The model under review builds one solid part; all positions refer to its coordinate system, in mm. Round coordinates to 2 decimals unless told otherwise and drop trailing zeros. Order: outer loops, then holes, each group sorted by start corner. A loop starts at its lowest first (then second) coordinate and runs counter-clockwise, first axis right, second up. Notation, with made-up numbers: (12.25, -22.5) -> (71.25, -22.5) arc R19 ccw to (71.25, 9.5) -> close; hole circle Ø6 at (33.25, 60.5). An arc over 180 degrees is marked (long way). Use a Markdown table: item, result. Add a question column.
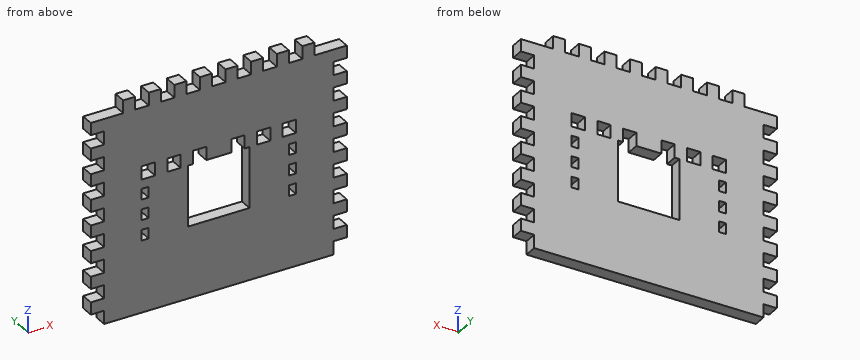
```python
from build123d import *

# Parameters (mm, degrees)
SKETCH1_W           = 127
SKETCH1_H           = 107.95
BOSS_EXTRUDE1_DEPTH = 6.35
SKETCH2_W           = 6.604
SKETCH2_H           = 6.604
CUT_EXTRUDE1_DEPTH  = 84.58153579
SKETCH3_W           = 3.429
SKETCH3_H           = 5.334
SKETCH3_W_2         = 6.604
SKETCH3_H_2         = 6.604
CUT_EXTRUDE4_DEPTH  = 84.58153579


with BuildPart() as part:
    # Sketch1 → Boss-Extrude1 (new body)
    with BuildSketch(Plane(origin=(0, 0, 0), x_dir=(1, 0, 0), z_dir=(0, 1, 0))):
        Rectangle(SKETCH1_W, SKETCH1_H)
    extrude(amount=BOSS_EXTRUDE1_DEPTH)

    # Sketch2 → Cut-Extrude1 (cut, through all)
    with BuildSketch(Plane.XZ):
        Polygon((-34.7345, 47.625), (-41.4655, 47.625), (-41.4655, 54.229), (-47.4345, 54.229), (-47.4345, 47.625), (-56.896, 47.625), (-63.5, 47.625), (-63.5, 54.229), (-63.5, 63.03162391), (63.5, 63.03162391), (63.5, 54.229), (63.5, 47.625), (56.896, 47.625), (47.4345, 47.625), (47.4345, 54.229), (41.4655, 54.229), (41.4655, 47.625), (34.7345, 47.625), (34.7345, 54.229), (28.7655, 54.229), (28.7655, 47.625), (22.0345, 47.625), (22.0345, 54.229), (16.0655, 54.229), (16.0655, 47.625), (9.3345, 47.625), (9.3345, 54.229), (3.3655, 54.229), (3.3655, 47.625), (-3.3655, 47.625), (-3.3655, 54.229), (-9.3345, 54.229), (-9.3345, 47.625), (-16.0655, 47.625), (-16.0655, 54.229), (-22.0345, 54.229), (-22.0345, 47.625), (-28.7655, 47.625), (-28.7655, 54.229), (-34.7345, 54.229), align=None)
        with Locations((60.198, 38.227)):
            Rectangle(SKETCH2_W, SKETCH2_H)
        with Locations((60.198, 25.527)):
            Rectangle(SKETCH2_W, SKETCH2_H)
        with Locations((60.198, 12.827)):
            Rectangle(SKETCH2_W, SKETCH2_H)
        with Locations((60.198, 0.127)):
            Rectangle(SKETCH2_W, SKETCH2_H)
        with Locations((60.198, -12.573)):
            Rectangle(SKETCH2_W, SKETCH2_H)
        with Locations((60.198, -25.273)):
            Rectangle(SKETCH2_W, SKETCH2_H)
        with Locations((60.198, -37.973)):
            Rectangle(SKETCH2_W, SKETCH2_H)
        with Locations((-60.198, -37.973)):
            Rectangle(SKETCH2_W, SKETCH2_H)
        with Locations((-60.198, -25.273)):
            Rectangle(SKETCH2_W, SKETCH2_H)
        with Locations((-60.198, -12.573)):
            Rectangle(SKETCH2_W, SKETCH2_H)
        with Locations((-60.198, 0.127)):
            Rectangle(SKETCH2_W, SKETCH2_H)
        with Locations((-60.198, 12.827)):
            Rectangle(SKETCH2_W, SKETCH2_H)
        with Locations((-60.198, 25.527)):
            Rectangle(SKETCH2_W, SKETCH2_H)
        with Locations((-60.198, 38.227)):
            Rectangle(SKETCH2_W, SKETCH2_H)
        with Locations((60.198, -50.673)):
            Rectangle(SKETCH2_W, SKETCH2_H)
        with Locations((-60.198, -50.673)):
            Rectangle(SKETCH2_W, SKETCH2_H)
    extrude(amount=-CUT_EXTRUDE1_DEPTH, mode=Mode.SUBTRACT)

    # Sketch3 → Cut-Extrude4 (cut, through all)
    with BuildSketch(Plane(origin=(0, 0, 0), x_dir=(1, 0, 0), z_dir=(0, 1, 0))):
        with Locations((-36.5125, 5.461)):
            Rectangle(SKETCH3_W, SKETCH3_H)
        Polygon((15.24, 18.288), (-15.24, 18.288), (-15.24, -11.938), (-12.827, -11.938), (-12.827, -18.542), (-6.223, -18.542), (-6.223, -11.938), (6.223, -11.938), (6.223, -18.542), (12.827, -18.542), (12.827, -11.938), (15.24, -11.938), align=None)
        with Locations((-36.5125, 15.621)):
            Rectangle(SKETCH3_W, SKETCH3_H)
        with Locations((-36.5125, -4.699)):
            Rectangle(SKETCH3_W, SKETCH3_H)
        with Locations((-22.225, -15.24)):
            Rectangle(SKETCH3_W_2, SKETCH3_H_2)
        with Locations((-34.925, -15.24)):
            Rectangle(SKETCH3_W_2, SKETCH3_H_2)
        with Locations((22.225, -15.24)):
            Rectangle(SKETCH3_W_2, SKETCH3_H_2)
        with Locations((34.925, -15.24)):
            Rectangle(SKETCH3_W_2, SKETCH3_H_2)
        with Locations((36.5125, -4.699)):
            Rectangle(SKETCH3_W, SKETCH3_H)
        with Locations((36.5125, 5.461)):
            Rectangle(SKETCH3_W, SKETCH3_H)
        with Locations((36.5125, 15.621)):
            Rectangle(SKETCH3_W, SKETCH3_H)
    extrude(amount=CUT_EXTRUDE4_DEPTH, mode=Mode.SUBTRACT)


solid = part.part
```
Q1. Add section A-A (x = -1). Write out the cut boundary in (y, z) (3 decimals), then the cut area to 3 significant figures.
Q2. Add section C-C (z = -26). Write out the cut boundary in (x, y), then the cut area to 3 significant figures.
Q3. Add section B-B (y = 1). State how many separate pieces and enclosed holes the cut face has, then the cut area to 3 significant figures.
Q4. Wall thickness on line 1 (X direction, y = 2, z = -18); line 2 (Z direction, x = -36, y = 4) (3 decimals); line 3 (X direction, y = 0.5, z = -14.5): over which ranges is each line inside the solid? List them lowest first. Write a range as [from, to].
Q5. Insertion check: pin 1 (1.9 mm diameter, centred on y = 4.5, z = -39.5, fed in from +X); pin 2 (2 mm diameter, centred on y = 5, z = -26.5, fed in from -X). Each pin has a flat end and moves straight along its axis. Give the tip position at first contact, or say it passes through.
Report:
| question | item | result |
|---|---|---|
| 1 | outline | (0, -53.975) -> (6.35, -53.975) -> (6.35, -18.288) -> (0, -18.288) -> close; (0, 11.938) -> (6.35, 11.938) -> (6.35, 47.625) -> (0, 47.625) -> close |
| 1 | area | 453 mm² |
| 2 | outline | (-56.9, 0) -> (56.9, 0) -> (56.9, 6.35) -> (-56.9, 6.35) -> close |
| 2 | area | 723 mm² |
| 3 | separate pieces | 1 |
| 3 | enclosed holes | 11 |
| 3 | area | 11,200 mm² |
| 4 | line 1 | x = [-63.5, -38.23], [-34.8, -15.24], [15.24, 34.8], [38.23, 63.5] |
| 4 | line 2 | z = [-53.975, -18.288], [-12.954, -8.128], [-2.794, 2.032], [7.366, 11.938], [18.542, 47.625] |
| 4 | line 3 | x = [-56.9, -38.23], [-34.8, -15.24], [15.24, 34.8], [38.23, 56.9] |
| 5 | pin 1 | stops at x = 56.9 |
| 5 | pin 2 | stops at x = -56.9 |
